Input: part model. Units: mm. Frame: model coordinates. Coordinates: 2 decimals unless noted, no trailing zeros. Order: outer loops, then holes, each group sorted by start corner. A loop starts at its lowest first (then second) coordinate and runs counter-clockwise, first axis right, second up. Notation, with made-up numbers: M -26,43.5 L 21,43.5 A30 cw 21,65.5 Z; hole C -20.5,-16.5 d1. An arc over 180 degrees is marked long. One line per item, written item: value.
Autodesk Inventor part; units mm, degrees
ref_plane "YZ Plane" through (0, 0, 0) normal (1, 0, 0) x (0, 1, 0)
ref_plane "XZ Plane" through (0, 0, 0) normal (0, 1, 0) x (-1, 0, 0)
ref_plane "XY Plane" through (0, 0, 0) normal (0, 0, 1) x (1, 0, 0)
sketch "Sketch1" plane through (0, 0, 0) normal (0, 0, 1) x (1, 0, 0)
  line L0 (0, 203.2) -> (0, 0)
  line L1 (0, 0) -> (-88.9, 0)
  line L2 (-175.9764, 101.6) -> (-175.9764, 87.0764)
  arc A0 (-175.9764, 87.0764) -> (-88.9, 0) centre (-88.9, 87.0764) ccw
  line L3 (-175.9764, 101.6) -> (0, 203.2)
  line L4 (0, -62.2809) -> (0, 247.4468)
  dimension "d1" = 203.2
  dimension "d2" = 60
  dimension "d3" = 203.2
  dimension "d4" = 88.9
extrude "Extrusion1" add sketch "Sketch1" along normal mid plane 381
properties part number "DMJ_Waist"
(1) Cut plane B-B on x = -61.5. Output: boundary loops of the cut face in (y, z).
Data:
outline: M 0,-190.5 L 167.69,-190.5 L 167.69,190.5 L 0,190.5 Z
(2) First-contact query: pin 1 (12 mm diameter, centred on y = 74.5, z = -142, fed in from -X); pin 2 (8 mm diameter, centred on x = -45.5, z = -44.5, fed in from +Y); pin 3 (5 mm diameter, centred on y = 80, z = 13.5, fed in from -X). Flat tips, straight axial feed; report the tip coordinate or a pass-through.
Data:
pin 1: stops at x = -175.73
pin 2: stops at y = 179.24
pin 3: stops at x = -175.86
(3) Cut plane A-A on z = 166.5. Output: boundary loops of the cut face in (x, y), plus the area to 3 significant figures.
Data:
outline: M -175.98,87.08 A87.08 ccw -88.9,0 L 0,0 L 0,203.2 L -175.98,101.6 Z
area: 25,200 mm2
(4) Ray query, line 1 (Y direction, x = -143, z = -166.5); line 2 (Y direction, x = -71, z = 127); line 3 (X direction, y = 180, z = -1). Return the intervals inside material, ascending. Write a range as from..to.
Data:
line 1: y = 18.85..120.64
line 2: y = 0..162.21
line 3: x = -40.18..0
(5) Cut plane C-C on y = 184.5. Output: boundary loops of the cut face in (x, z).
Data:
outline: M -32.39,-190.5 L 0,-190.5 L 0,190.5 L -32.39,190.5 Z
